```python
from build123d import *

# Parameters (mm, degrees)
F1_DEPTH = 18
F2_W     = 25.921413
F2_H     = 7.5
F3_DEPTH = 25
F4_R     = 2
F5_DEPTH = 25


with BuildPart() as f1:
    # F0 (on Front) → F1 (new body)
    with BuildSketch(Plane.XZ):
        with BuildLine():
            Line((-20, 0), (0, 0))
            Line((0, 0), (20, 0))
            ThreePointArc((20, 0), (24.300527, 3.175061), (22.532417, 8.219794))
            Line((22.532417, 8.219794), (6, 19.474979))
            Line((6, 19.474979), (-6, 19.474979))
            Line((-6, 19.474979), (-22.532417, 8.219794))
            ThreePointArc((-22.532417, 8.219794), (-24.300527, 3.175061), (-20, 0))
        make_face()
    extrude(amount=F1_DEPTH)

    # F2 (on face) → F3 (cut)
    with BuildSketch(Plane.XY.offset(19.474979)):
        with Locations((-18.960707, -9)):
            Rectangle(F2_W, F2_H)
        with Locations((18.960707, -9)):
            Rectangle(F2_W, F2_H)
    extrude(amount=-F3_DEPTH, mode=Mode.SUBTRACT)

    # F4 (on face) → F5 (cut)
    with BuildSketch(Plane.XZ.offset(18)):
        with Locations((-20, 4.5)):
            Circle(F4_R)
        with Locations((20, 4.5)):
            Circle(F4_R)
    extrude(amount=-F5_DEPTH, mode=Mode.SUBTRACT)


solid = f1.part
```
CAD build for the part. Positions are in the model's coordinates, mm. A direction names the side the tool comes from. Round coordinates to 2 decimals unless told otherwise and drop trailing zeros. Write each loop counter-clockwise with the first axis right and the second up, starting at its lowest first coordinate (ties: lowest second). Pieces come first, ordered by that corner, then holes. Notation, with made-up numbers: (60.25, -17) - (83.25, -17) arc R17 cw to (83.25, -8) - close; hole circle Ø1 at (49.5, -25). An arc over 180 degrees is marked (long way). Return JSON: item names as keys, results as strings. Group by question number.
Item 1: Band-saw the part on D-D on z = 13.25. List the corners of the cut face in (x, y), plus the area to 3 significant figures.
Item 2: Mould opens along Y. For faces 1 (the face through (0, -18, 8)), 2 (the face through (0, 0, 8)), 3 (the face through (6, -9, 10)), 4 (the face through (0, -9, 19.475)) say: +Y half, -Y half, draft (parallel to the pull), parting line (faces both ways), or undercut.
Item 3: Flat gauge pins, fed straight in: pin 1 Ø2 at (y, z) = (-10, 14.5) entering from +X; pin 2 Ø1 at (x, y) = (11.5, -4.5) entering from +Z; pin 3 Ø6 at (y, z) = (-4.5, 14) entering from +X. Where does each tip first touch, or does it go through?
Item 4: 3-axis set-ups, long thin cutter, end or side, ignore diameter. For faces 5 (the face through (13, -5.25, 8)), 6 (the face through (-13, -12.75, 8)), 7 (the face through (-24.323, -2.588, 3.252)): which of +Z, -Z, +X, -X, +Y, -Y reach the whole face in a straight line?
Item 5: Band-saw the part on C-C on x = -11. List the corners of the cut face in (y, z).
Item 6: Band-saw the part on B-B on y = -4.5. List the corners of the cut face in (x, z), plus the area to 3 significant figures.
Item 7: Probe probe 1 along Y at (x, z) = (-12, 4); probe 2 along X at (y, z) = (-1, 5.5); probe 3 along Z at (x, y) = (20, -14.4). List the from-to ranges inside material, lowest first.
Item 8: Band-saw the part on A-A on z = 4.5. List the corners of the cut face in (x, y), plus the area to 4 significant figures.
Resolved:
{
 "1": {"outline": "(-15.14, -18) - (15.14, -18) - (15.14, -12.75) - (6, -12.75) - (6, -5.25) - (15.14, -5.25) - (15.14, 0) - (-15.14, 0) - (-15.14, -5.25) - (-6, -5.25) - (-6, -12.75) - (-15.14, -12.75) - close", "area": "408 mm²"},
 "2": {"face 1": "-Y half", "face 2": "+Y half", "face 3": "undercut", "face 4": "draft"},
 "3": {"pin 1": "stops at x = 6", "pin 2": "stops at z = 16.07", "pin 3": "stops at x = 18.45"},
 "4": {"face 5": "+Z, -Z, +X", "face 6": "+Z, -Z, -X", "face 7": "-X, +Y, -Y"},
 "5": {"outline": "(-18, 0) - (-12.75, 0) - (-12.75, 16.07) - (-18, 16.07) - close; (-5.25, 0) - (0, 0) - (0, 16.07) - (-5.25, 16.07) - close"},
 "6": {"outline": "(-22.53, 8.22) arc R4.5 ccw to (-20, 0) - (20, 0) arc R4.5 ccw to (22.53, 8.22) - (6, 19.47) - (-6, 19.47) - close; hole circle Ø4 at (-20, 4.5); hole circle Ø4 at (20, 4.5)", "area": "686 mm²"},
 "7": {"probe 1": "y = -18 to -12.75, -5.25 to 0", "probe 2": "x = -24.39 to -21.73, -18.27 to 18.27, 21.73 to 24.39", "probe 3": "z = 0 to 2.5, 6.5 to 9.94"},
 "8": {"outline": "(-24.5, -18) - (-22, -18) - (-22, -12.75) - (-24.5, -12.75) - close; (-24.5, -5.25) - (-22, -5.25) - (-22, 0) - (-24.5, 0) - close; (-18, -18) - (18, -18) - (18, -12.75) - (6, -12.75) - (6, -5.25) - (18, -5.25) - (18, 0) - (-18, 0) - (-18, -5.25) - (-6, -5.25) - (-6, -12.75) - (-18, -12.75) - close; (22, -18) - (24.5, -18) - (24.5, -12.75) - (22, -12.75) - close; (22, -5.25) - (24.5, -5.25) - (24.5, 0) - (22, 0) - close", "area": "520.5 mm²"}
}
